from build123d import *

# Parameters (mm, degrees)
SKETCH_1_R          = 12.5
EXTRUDE_2_DEPTH     = 235.43
SKETCH_2_R          = 9
CUT_EXTRUDE_1_DEPTH = 235.43
EXTRUDE_START       = 15.57
SKETCH_3_R          = 12.5
EXTRUDE_3_DEPTH     = 15.57
SKETCH_4_R          = 9
CUT_EXTRUDE_2_DEPTH = 20
EXTRUDE_START_2     = 9.93
SKETCH_5_R          = 12.5
EXTRUDE_4_DEPTH     = 9.93
SKETCH_6_R          = 9
CUT_EXTRUDE_3_DEPTH = 10
SKETCH_7_R          = 26.85848727
CUT_EXTRUDE_4_DEPTH = 14.93
SKETCH_8_R          = 12.5
EXTRUDE_5_DEPTH     = 9.93
SKETCH_9_R          = 9
CUT_EXTRUDE_5_DEPTH = 10
SKETCH_10_R         = 37.193394561
CUT_EXTRUDE_6_DEPTH = 0.22
SKETCH_11_R         = 43.187188263
CUT_EXTRUDE_7_DEPTH = 0.71
SKETCH_12_R         = 12.5
EXTRUDE_6_DEPTH     = 15
CUT_EXTRUDE_START   = -15
SKETCH_13_R         = 9
CUT_EXTRUDE_8_DEPTH = 15
SKETCH_14_R         = 11
CUT_EXTRUDE_9_DEPTH = 320


with BuildPart() as part:
    # 草图1 → 凸台-拉伸2 (new body)
    with BuildSketch(Plane.XY):
        Circle(SKETCH_1_R)
    extrude(amount=EXTRUDE_2_DEPTH)

    # 草图2 → 切除-拉伸1 (cut)
    with BuildSketch(Plane(origin=(0, 0, 0), x_dir=(-1, 0, 0), z_dir=(0, 0, -1))):
        Circle(SKETCH_2_R)
    extrude(amount=-CUT_EXTRUDE_1_DEPTH, mode=Mode.SUBTRACT)

    # 草图3 → 凸台-拉伸3 (add)
    with BuildSketch(Plane(origin=(0, 0, 0), x_dir=(-1, 0, 0), z_dir=(0, 0, -1)).offset(EXTRUDE_START)):
        Circle(SKETCH_3_R)
    extrude(amount=-EXTRUDE_3_DEPTH)

    # 草图4 → 切除-拉伸2 (cut)
    with BuildSketch(Plane(origin=(0, 0, -15.57), x_dir=(-1, 0, 0), z_dir=(0, 0, -1))):
        Circle(SKETCH_4_R)
    extrude(amount=-CUT_EXTRUDE_2_DEPTH, mode=Mode.SUBTRACT)

    # 草图5 → 凸台-拉伸4 (add)
    with BuildSketch(Plane(origin=(0, 0, -15.57), x_dir=(-1, 0, 0), z_dir=(0, 0, -1)).offset(EXTRUDE_START_2)):
        Circle(SKETCH_5_R)
    extrude(amount=-EXTRUDE_4_DEPTH)

    # 草图6 → 切除-拉伸3 (cut)
    with BuildSketch(Plane(origin=(0, 0, -25.5), x_dir=(-1, 0, 0), z_dir=(0, 0, -1))):
        Circle(SKETCH_6_R)
    extrude(amount=-CUT_EXTRUDE_3_DEPTH, mode=Mode.SUBTRACT)

    # 草图7 → 切除-拉伸4 (cut)
    with BuildSketch(Plane(origin=(0, 0, -25.5), x_dir=(-1, 0, 0), z_dir=(0, 0, -1))):
        Circle(SKETCH_7_R)
    extrude(amount=-CUT_EXTRUDE_4_DEPTH, mode=Mode.SUBTRACT)

    # 草图8 → 凸台-拉伸5 (add)
    with BuildSketch(Plane(origin=(0, 0, -10.57), x_dir=(-1, 0, 0), z_dir=(0, 0, -1)).offset(EXTRUDE_START_2)):
        Circle(SKETCH_8_R)
    extrude(amount=-EXTRUDE_5_DEPTH)

    # 草图9 → 切除-拉伸5 (cut)
    with BuildSketch(Plane(origin=(0, 0, -20.5), x_dir=(-1, 0, 0), z_dir=(0, 0, -1))):
        Circle(SKETCH_9_R)
    extrude(amount=-CUT_EXTRUDE_5_DEPTH, mode=Mode.SUBTRACT)

    # 草图10 → 切除-拉伸6 (cut)
    with BuildSketch(Plane(origin=(0, 0, -20.5), x_dir=(-1, 0, 0), z_dir=(0, 0, -1))):
        with Locations((7.201744855, 7.507888779)):
            Circle(SKETCH_10_R)
    extrude(amount=-CUT_EXTRUDE_6_DEPTH, mode=Mode.SUBTRACT)

    # 草图11 → 切除-拉伸7 (cut)
    with BuildSketch(Plane(origin=(0, 0, -20.28), x_dir=(-1, 0, 0), z_dir=(0, 0, -1))):
        with Locations((-1.225460352, 2.329416421)):
            Circle(SKETCH_11_R)
    extrude(amount=-CUT_EXTRUDE_7_DEPTH, mode=Mode.SUBTRACT)

    # 草图12 → 凸台-拉伸6 (add)
    with BuildSketch(Plane.XY.offset(235.43)):
        with Locations(Location((0, 0, 0), (0, 0, 180))):
            Circle(SKETCH_12_R)
    extrude(amount=EXTRUDE_6_DEPTH)

    # 草图13 → 切除-拉伸8 (cut)
    with BuildSketch(Plane.XY.offset(250.43).offset(CUT_EXTRUDE_START)):
        with Locations(Location((0, 0, 0), (0, 0, 180))):
            Circle(SKETCH_13_R)
    extrude(amount=CUT_EXTRUDE_8_DEPTH, mode=Mode.SUBTRACT)

    # 草图14 → 切除-拉伸9 (cut)
    with BuildSketch(Plane(origin=(0, 0, -19.57), x_dir=(-1, 0, 0), z_dir=(0, 0, -1))):
        Circle(SKETCH_14_R)
    extrude(amount=-CUT_EXTRUDE_9_DEPTH, mode=Mode.SUBTRACT)


solid = part.part
The model under review builds one solid part; all positions refer to its coordinate system, in mm. Round coordinates to 2 decimals unless told otherwise and drop trailing zeros. Write each loop counter-clockwise with the first axis right and the second up, starting at its lowest first coordinate (ties: lowest second). Pieces come first, ordered by that corner, then holes. Notation, with made-up numbers: M 64,85.5 L 116,85.5 A17 cw 116,116.5 Z; hole C -31.75,-25 d10. An arc over 180 degrees is marked long. Answer as CSV lines item,"result". Start each with the question number.
Q1. Clearance check with flat-ended pins moving along their axes: P1, Ø2, axis at y = -8, z = 189, coming from the -X side; P2, Ø6, axis at y = 4, z = 87, coming from the -X side; P3, Ø4, axis at x = -7.5, z = 113.5, coming from the +Y side (3 decimals); P4, Ø6, axis at x = 1, z = 75.5, coming from the -Y side. State where each tip first meets the part, or that it passes through.
Q2. The part is to be moulded in two halves that separate along Y. For faces 1 (the face through (-5, 10, 250.43)), 2 (the face through (2.38, -10.74, 113.54)), say which applies: +Y half, -Y half, draft (parallel to the pull), parting line (faces both ways), or undercut.
Q3. Consider section C-C, the plane z = 63. Give the boundary of the cut face in (x, y), then the cut area to 3 significant figures.
Q4. Consider section A-A, the plane y = 0. Give the boundary of the cut face in (x, z).
Q5. Wall thickness on line 1 along Y through (x, z) = (0, 174.5); line 2 along X through (y, z) = (-1, 148.5); line 3 along X through (y, z) = (-8, 154.5): over which ranges is each line inside the solid? List them lowest first.
Result set:
1,P1,"stops at x = -10.36"
1,P2,"stops at x = -12.46"
1,P3,"stops at y = 11.225"
1,P4,"stops at y = -12.5"
2,face 1,"draft"
2,face 2,"undercut"
3,outline,"C 0,0 d25; hole C 0,0 d22"
3,area,"111 mm²"
4,outline,"M -12.5,-19.57 L -11,-19.57 L -11,250.43 L -12.5,250.43 Z; M 11,-19.57 L 12.5,-19.57 L 12.5,250.43 L 11,250.43 Z"
5,line 1,"y = -12.5 to -11, 11 to 12.5"
5,line 2,"x = -12.46 to -10.95, 10.95 to 12.46"
5,line 3,"x = -9.6 to -7.55, 7.55 to 9.6"
